```python
from build123d import *

# Parameters (mm, degrees)
BOSS_EXTRUDE1_DEPTH = 25
CUT_EXTRUDE1_DEPTH  = 25
BOSS_EXTRUDE2_DEPTH = 15


with BuildPart() as part:
    # Sketch1 → Boss-Extrude1 (new body)
    with BuildSketch(Plane.XY):
        Polygon((-30, 10), (-15, 10), (-15, 25), (0, 25), (0, 0), (-30, 0), align=None)
    extrude(amount=BOSS_EXTRUDE1_DEPTH)

    # Sketch2 → Cut-Extrude1 (cut)
    with BuildSketch(Plane.ZY.offset(15)):
        Polygon((0, 10), (25, 25), (0, 25), align=None)
    extrude(amount=-CUT_EXTRUDE1_DEPTH, mode=Mode.SUBTRACT)

    # Sketch4 → Boss-Extrude2 (add)
    with BuildSketch(Plane.ZY.offset(15)):
        Polygon((25, 10), (0, 10), (0, 25), align=None)
    extrude(amount=BOSS_EXTRUDE2_DEPTH)


solid = part.part
```
Source: CAD feature listing. Evaluate the final solid. Frame: model axes, mm. A direction names the side the tool comes from. Coordinates: 2 decimals unless noted, no trailing zeros. Write each loop counter-clockwise with the first axis right and the second up, starting at its lowest first coordinate (ties: lowest second). Pieces come first, ordered by that corner, then holes. Notation, with made-up numbers: M -17,83 L 16,83 A10 ccw 16,101 Z; hole C 22,32.25 d7. An arc over 180 degrees is marked long. Answer as a JSON object with one key per item and string values.
1. Ray query, L1, parallel to X at y = 22.25, z = 2.75; L2, parallel to X at y = 17.5, z = 17.25; L3, parallel to Y at x = -13, z = 5.75. Return the intervals inside material, ascending.
Evaluation:
{"L1": "-30 to -15", "L2": "-15 to 0", "L3": "0 to 13.45"}
2. Contact query for flat-ended pins moving along their axis: P1, Ø12, axis at x = -10.5, y = 18, coming from the -Z side; P2, Ø3, axis at x = -24.5, z = 13, coming from the +Y side. Output: stop coordinate, or through.
Evaluation:
{"P1": "z = 0", "P2": "y = 18.1"}
3. Access query for faces 1 (the flat face through (-15, 18, 5)), 2 (the flat face through (-18, 10, 0)), 3 (the flat face through (-22.395, 17.605, 12.325)). Directions: +Z, -Z, +X, -X, +Y, -Y. A direction counts if a zero-diameter tool reaches every point of the face in a straight line with its end or side. Return the directions, or none.
Evaluation:
{"face 1": "-Z, +X, +Y", "face 2": "-Z, +X, -X, +Y, -Y", "face 3": "+Z, -X, +Y"}
4. Cut plane D-D on y = 20.75. Output: boundary loops of the cut face in (x, z).
Evaluation:
{"outline": "M -30,0 L -15,0 L -15,7.08 L -30,7.08 Z; M -15,17.92 L 0,17.92 L 0,25 L -15,25 Z"}
5. Cut plane C-C on x = -5. Output: boundary loops of the cut face in (y, z).
Evaluation:
{"outline": "M 0,0 L 10,0 L 25,25 L 0,25 Z"}
6. Cut plane A-A on y = 18. Output: boundary loops of the cut face in (x, z), plus the area to 3 significant figures.
Evaluation:
{"outline": "M -30,0 L -15,0 L -15,11.67 L -30,11.67 Z; M -15,13.33 L 0,13.33 L 0,25 L -15,25 Z", "area": "350 mm^2"}
7. Cut plane B-B on z = 5.5. Output: boundary loops of the cut face in (x, y), plus the area to 3 significant figures.
Evaluation:
{"outline": "M -30,0 L 0,0 L 0,13.3 L -15,13.3 L -15,21.7 L -30,21.7 Z", "area": "525 mm^2"}
